Geometry: final body of the model. Coordinates: model frame, mm. Face numbers are marked on the shaded views. A direction names the side the tool comes from. Coordinates: 2 decimals unless noted, no trailing zeros. Write each loop counter-clockwise with the first axis right and the second up, starting at its lowest first coordinate (ties: lowest second). Pieces come first, ordered by that corner, then holes. Notation, with made-up numbers: (76.25, 87.5) - (116.25, 87.5) arc R31 ccw to (116.25, 119.5) - close; hole circle Ø8 at (-10, -4). An arc over 180 degrees is marked (long way). Answer as a JSON object with one key per item and string values. Group by question number.
Item 1: Section C-C on z = 55.88. Return loops of the section in (x, y).
Item 2: Section D-D on z = -82. Return loops of the section in (x, y) (3 decimals), and give its area (3 significant figures).
Item 3: Section A-A on y = 19.05. State how many separate pieces and enclosed holes the cut face has, and give its area (3 significant figures).
Item 4: Line query: line 1 along X through (y, z) = (28, 55.88); line 2 along Z through (x, y) = (-73, 12); line 3 along Z through (x, y) = (-9.5, -2). Output: solid intervals per line, ascending. Write a range as from..to.
Item 5: Set-up query: the marked faces 1, 2 and 3. Return all of +Z, -Z, +X, -X, +Y, -Y with unobstructed straight access to the full face (end or side cutting, diameter ignored); none if empty.
Item 6: Mould query, pull axis X, two halves, no side actions, for the marked faces 4, 5, 6 and 7. Classes: pulls with the +X half, pulls with the -X half, needs draft (parallel to the pull), parting line crosses it, or undercut.
Item 7: First-contact query: pin 1 Ø2 at (y, z) = (10, -31) entering from -X; pin 2 Ø25 at (x, z) = (-22, -47) entering from +Y; pin 3 Ø3 at (x, z) = (-55.5, -28) entering from +Y; pin 4 Ø16 at (x, z) = (-42.5, 58) entering from -Y. Flat tips, straight axial feed; report the tip coordinate or a pass-through.
```python
from build123d import *

# Parameters (mm, degrees)
SKETCH2_R           = 15.875
BOSS_EXTRUDE1_DEPTH = 82.55
SKETCH4_R           = 7.9375
CUT_EXTRUDE1_DEPTH  = 144.384968543
SKETCH5_R           = 19.304
CUT_EXTRUDE2_DEPTH  = 191.634403254


with BuildPart() as part:
    # Sketch2 → Boss-Extrude1 (new body)
    with BuildSketch(Plane(origin=(0, 0, 0), x_dir=(0, 0, -1), z_dir=(1, 0, 0))):
        with BuildLine():
            ThreePointArc((0, -31.75), (-26.563955842, -17.390191201), (-29.099355663, 12.7))
            Line((-29.099355663, 12.7), (-82.55, 12.7))
            Line((-82.55, 12.7), (-82.55, 31.75))
            Line((-82.55, 31.75), (0, 31.75))
            ThreePointArc((0, 31.75), (26.563955842, 17.390191201), (29.099355663, -12.7))
            Line((29.099355663, -12.7), (79.502, -12.7))
            Line((79.502, -12.7), (79.502, 57.15))
            Line((79.502, 57.15), (98.552, 57.15))
            Line((98.552, 57.15), (98.552, -31.75))
            Line((98.552, -31.75), (0, -31.75))
        make_face()
        Circle(SKETCH2_R, mode=Mode.SUBTRACT)
    extrude(amount=-BOSS_EXTRUDE1_DEPTH)

    # Sketch4 → Cut-Extrude1 (cut, through all)
    with BuildSketch(Plane(origin=(0, 31.75, 0), x_dir=(1, 0, 0), z_dir=(0, 1, 0))):
        with Locations(Location((-63.5, -55.88, 0), (0, 0, 270))):
            Circle(SKETCH4_R)
        with Locations(Location((-19.05, -55.88, 0), (0, 0, 270))):
            Circle(SKETCH4_R)
    extrude(amount=-CUT_EXTRUDE1_DEPTH, mode=Mode.SUBTRACT)

    # Sketch5 → Cut-Extrude2 (cut, through all)
    with BuildSketch(Plane.XY.offset(-79.502)):
        Polygon((-82.55, 31.75), (-57.15, 57.15), (-82.55, 57.15), align=None)
        Polygon((-25.4, 57.15), (0, 31.75), (0, 57.15), align=None)
        with Locations((-41.275, 19.05)):
            Circle(SKETCH5_R)
    extrude(amount=-CUT_EXTRUDE2_DEPTH, mode=Mode.SUBTRACT)


solid = part.part
```
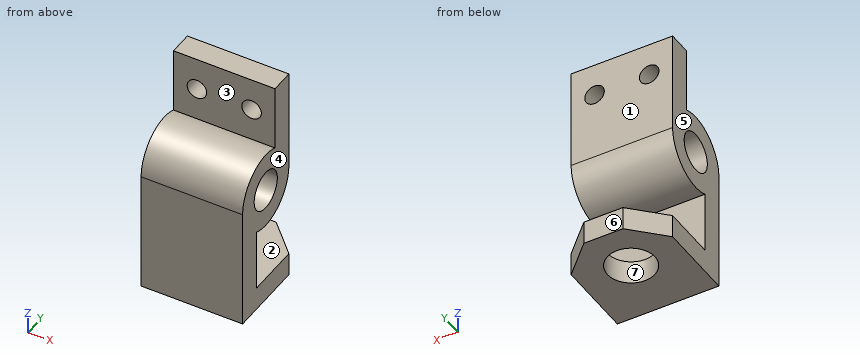
Checks:
{
 "1": {"outline": "(-82.55, 12.7) - (-71.44, 12.7) - (-71.44, 31.75) - (-82.55, 31.75) - close; (-55.56, 12.7) - (-26.99, 12.7) - (-26.99, 31.75) - (-55.56, 31.75) - close; (-11.11, 12.7) - (0, 12.7) - (0, 31.75) - (-11.11, 31.75) - close"},
 "2": {"outline": "(-82.55, -31.75) - (0, -31.75) - (0, 31.75) - (-25.4, 57.15) - (-57.15, 57.15) - (-82.55, 31.75) - close; hole circle Ø38.608 at (-41.275, 19.05)", "area": "5,520 mm^2"},
 "3": {"separate pieces": "3", "enclosed holes": "2", "area": "9,350 mm^2"},
 "4": {"line 1": "-82.55..-71.44, -55.56..-26.99, -11.11..0", "line 2": "-98.55..-79.5, -29.39..-10.39, 10.39..29.39", "line 3": "-98.55..-79.5, -31.69..-15.75, 15.75..31.69"},
 "5": {"face 1": "+Z, +X, -X, +Y", "face 2": "+X, -X, +Y", "face 3": "+Z, +X, -X"},
 "6": {"face 4": "pulls with the +X half", "face 5": "pulls with the -X half", "face 6": "needs draft", "face 7": "undercut"},
 "7": {"pin 1": "x = -82.55", "pin 2": "y = -12.7", "pin 3": "y = 17.49", "pin 4": "y = 12.7"}
}
